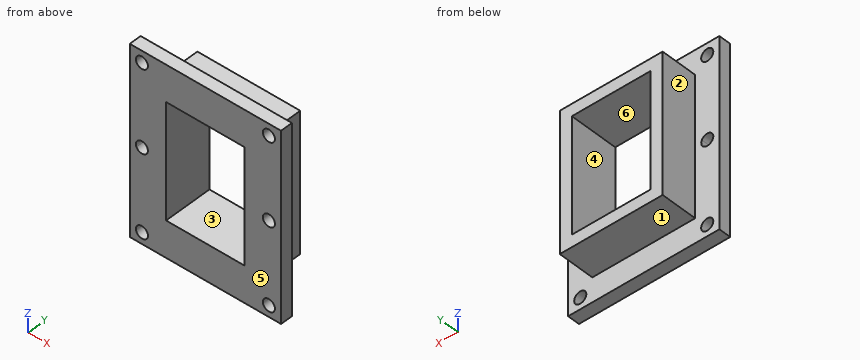
Autodesk Inventor part; units mm, degrees
ref_plane "YZ Plane" through (0, 0, 0) normal (1, 0, 0) x (0, 1, 0)
ref_plane "XZ Plane" through (0, 0, 0) normal (0, 1, 0) x (-1, 0, 0)
ref_plane "XY Plane" through (0, 0, 0) normal (0, 0, 1) x (1, 0, 0)
sketch "Sketch1" plane through (0, 0, 0) normal (0, 1, 0) x (-1, 0, 0)
  line L0 (-6.5, -9.5) -> (6.5, -9.5)
  line L1 (6.5, -9.5) -> (6.5, 9.5)
  line L2 (6.5, 9.5) -> (-6.5, 9.5)
  line L3 (-6.5, 9.5) -> (-6.5, -9.5)
  line L4 (-6.5, -9.5) -> (6.5, 9.5) construction
  line L5 (6.5, -9.5) -> (-6.5, 9.5) construction
  line L6 (-8.5, -11.5) -> (8.5, -11.5)
  line L7 (8.5, -11.5) -> (8.5, 11.5)
  line L8 (8.5, 11.5) -> (-8.5, 11.5)
  line L9 (-8.5, 11.5) -> (-8.5, -11.5)
  line L10 (-8.5, -11.5) -> (8.5, 11.5) construction
  line L11 (8.5, -11.5) -> (-8.5, 11.5) construction
  point P0 (0, 0)
  dimension "d0" = 13
  dimension "d1" = 19
  dimension "d2" = 17
  dimension "d3" = 23
extrude "Extrusion1" add sketch "Sketch1" along normal blind 8
sketch "Sketch2" plane through (0, 0, 0) normal (0, -1, 0) x (1, 0, 0)
  line L0 (8.5, 11.5) -> (8.5, -11.5)
  line L1 (-8.5, 11.5) -> (8.5, 11.5)
  line L2 (-8.5, -11.5) -> (-8.5, 11.5)
  line L3 (8.5, -11.5) -> (-8.5, -11.5)
  line L4 (-6.5, 9.5) -> (-6.5, -9.5)
  line L5 (6.5, 9.5) -> (-6.5, 9.5)
  line L6 (6.5, -9.5) -> (6.5, 9.5)
  line L7 (-6.5, -9.5) -> (6.5, -9.5)
  line L8 (-6.5, 9.5) -> (-6.5, -9.5)
  line L9 (6.5, 9.5) -> (-6.5, 9.5)
  line L10 (-6.5, 9.5) -> (-6.5, -9.5)
  line L11 (-6.5, -9.5) -> (6.5, -9.5)
  line L12 (6.5, -9.5) -> (6.5, 9.5)
  line L13 (6.5, 9.5) -> (-6.5, 9.5)
  line L14 (-6.5, -9.5) -> (6.5, -9.5)
  line L15 (6.5, -9.5) -> (6.5, 9.5)
  line L16 (6.5, 0) -> (12.5, 0)
  line L17 (12.5, 15.5) -> (-12.5, 15.5)
  line L18 (-12.5, 15.5) -> (-12.5, -15.5)
  line L19 (-12.5, -15.5) -> (12.5, -15.5)
  line L20 (12.5, -15.5) -> (12.5, 15.5)
  point P0 (0, 0)
  dimension "d9" = 25
extrude "Extrusion2" add sketch "Sketch2" against normal blind 2 contours L20 L19 L18 L17
sketch "Sketch3" plane through (0, 2, 0) normal (0, 1, 0) x (1, 0, 0)
  circle A0 centre (-10.4906, -13.5807) radius 1
  circle A1 centre (-10.5, 0) radius 1
  line L0 (-12.5, 15.5) -> (-12.5, -15.5)
  line L1 (-12.5, -15.5) -> (-12.5, 15.5)
  line L2 (-12.5, -15.5) -> (12.5, -15.5)
  circle A2 centre (-10.4906, 0.0193) radius 1
  circle A3 centre (-10.4906, 13.6193) radius 1
  line L3 (12.5, 15.5) -> (-12.5, 15.5)
  circle A4 centre (10.4906, -13.5807) radius 1
  circle A5 centre (10.4906, 0.0193) radius 1
  circle A6 centre (10.4906, 13.6193) radius 1
  point P0 (0, 0)
  point P1 (-11.3944, 0.4472)
  point P2 (-9.5962, -0.4279)
  dimension "d12" = 2
  dimension "d20" = 13.6
extrude "Extrusion3" cut sketch "Sketch3" against normal blind 2 contours A0 | A1 A2 | A3 | A4 | A5 | A6 picked at (-10.303, 0.2798)
properties part number "TipkaloDrzac_v.1.0"
Verification items for the finished model (mm, model axes). Face numbers are marked on the shaded views. A direction names the side the tool comes from. Give positions to 0.01 mm unless a question says otherwise; leave off trailing zeros. Order: outer loops, then holes, each group sorted by start corner. A loop starts at its lowest first (then second) coordinate and runs counter-clockwise, first axis right, second up. Notation, with made-up numbers: M -40,73.5 L -32,73.5 A13 cw -32,86.5 Z; hole C 60,27 d11. An arc over 180 degrees is marked long. Answer as a JSON object with one key per item and string values. Group by question number.
1) Cross-section at B-B (z = 1.5). Enter the section's corners in (x, y).
2) Mould release check, pull along Z, two halves, no side actions. Record for the marked faces 1, 2, 3 and 4: released by +Z, released by -Z, zero draft, split by the parting line, or undercut.
3) Scan lines: line 1 along Z through (x, y) = (-6, 7); line 2 along X through (y, z) = (4, -7); line 3 along Z through (x, y) = (-3.5, 1). Record each from-to range of solid material in increasing order. Write a range as [from, to].
4) Depth check by flat-ended pin: pin 1 Ø3 at (x, y) = (9, 7) entering from -Z; pin 2 Ø1.8 at (y, z) = (6.5, 1) entering from -X; pin 3 Ø1.6 at (x, z) = (10.49, -0.02) entering from +Y; pin 4 Ø1 at (y, z) = (5.5, 7) entering from +X. Enter the tip coordinate at first touch or a pass-through.
5) Cross-section at A-A (y = 3.5). Enter the section's corners in (x, z).
6) Cross-section at C-C (x = 0.25). Enter the section's corners in (y, z), then the cut area to 3 significant figures.
7) Access from +Z, -Z, +X, -X, +Y, -Y to the whole of each face (thin tool, end or side, straight path). Record for the marked faces 5 and 6.
8) Cross-section at D-D (x = -10.5). Enter the section's corners in (y, z), then the cut area to 3 significant figures.
Result sheet:
{
 "1": {"outline": "M -12.5,0 L -6.5,0 L -6.5,8 L -8.5,8 L -8.5,2 L -12.5,2 Z; M 6.5,0 L 12.5,0 L 12.5,2 L 8.5,2 L 8.5,8 L 6.5,8 Z"},
 "2": {"face 1": "released by -Z", "face 2": "zero draft", "face 3": "undercut", "face 4": "undercut"},
 "3": {"line 1": "z = [-11.5, -9.5], [9.5, 11.5]", "line 2": "x = [-8.5, -6.5], [6.5, 8.5]", "line 3": "z = [-15.5, -9.5], [9.5, 15.5]"},
 "4": {"pin 1": "stops at z = -11.5", "pin 2": "stops at x = -8.5", "pin 3": "passes through", "pin 4": "stops at x = 8.5"},
 "5": {"outline": "M -8.5,-11.5 L 8.5,-11.5 L 8.5,11.5 L -8.5,11.5 Z; hole M -6.5,-9.5 L 6.5,-9.5 L 6.5,9.5 L -6.5,9.5 Z"},
 "6": {"outline": "M 0,-15.5 L 2,-15.5 L 2,-11.5 L 8,-11.5 L 8,-9.5 L 0,-9.5 Z; M 0,9.5 L 8,9.5 L 8,11.5 L 2,11.5 L 2,15.5 L 0,15.5 Z", "area": "48.0 mm2"},
 "7": {"face 5": "+Z, -Z, +X, -X, -Y", "face 6": "+Y, -Y"},
 "8": {"outline": "M 0,-15.5 L 2,-15.5 L 2,-14.62 L 0,-14.62 Z; M 0,-12.62 L 2,-12.62 L 2,-1 L 0,-1 Z; M 0,0.98 L 2,0.98 L 2,12.58 L 0,12.58 Z; M 0,14.58 L 2,14.58 L 2,15.5 L 0,15.5 Z", "area": "50.0 mm2"}
}
